Job drawing, mm, ordinate dimensions from the low corner. One solid piece. Coordinates: 2 decimals unless noted, no trailing zeros. Order: outer loops, then holes, each group sorted by start corner. A loop starts at its lowest first (then second) coordinate and runs counter-clockwise, first axis right, second up. Notation, with made-up numbers: M -16.5,18 L 33.5,18 A20 ccw 33.5,49 Z; hole C 58,-9.75 d7. An arc over 180 degrees is marked long. Write item = value, one per line.
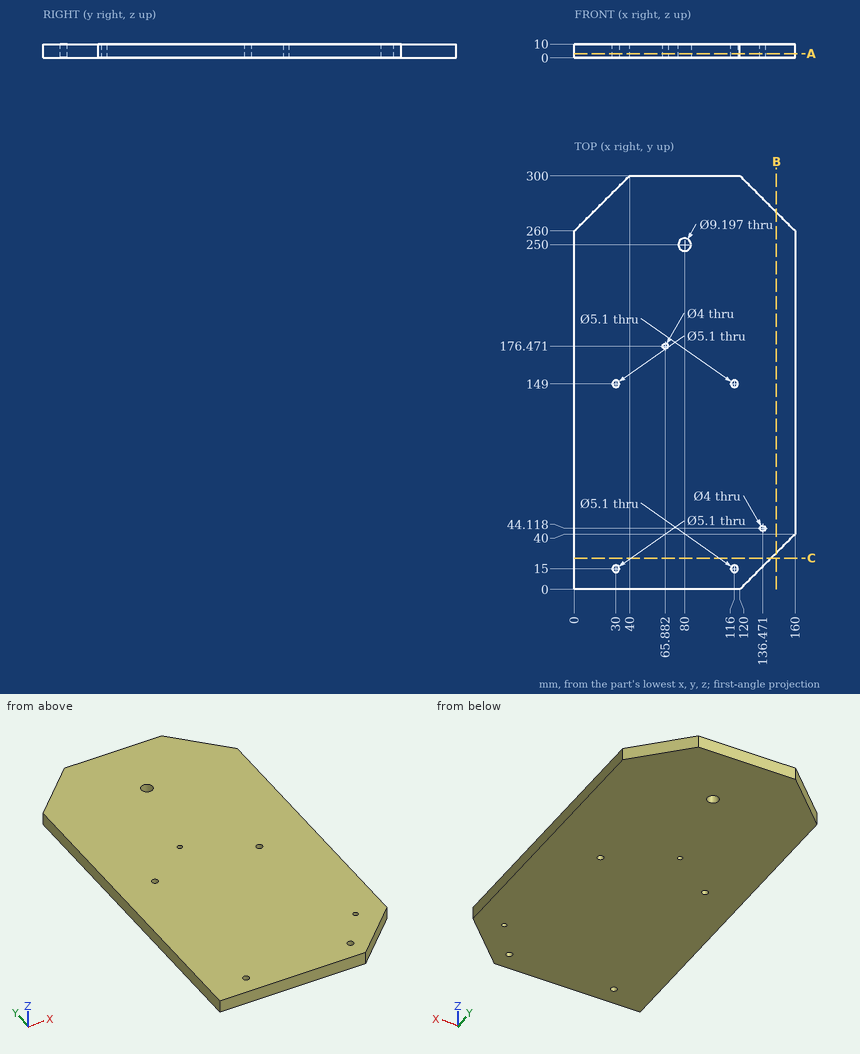
(1) Slice it at B-B, the plane x = 146.5. Write the cut outline in (y, z), then the cut area to 3 significant figures.
Evaluation:
outline = M 26.5,0 L 273.5,0 L 273.5,10 L 26.5,10 Z
area = 2,470 mm²
(2) Slice it at A-A, the plane z = 3. Write the cut outline in (x, y).
Evaluation:
outline = M 0,0 L 120,0 L 160,40 L 160,260 L 120,300 L 40,300 L 0,260 Z; hole C 30,15 d5.1; hole C 30,149 d5.1; hole C 65.88,176.47 d4; hole C 80,250 d9.2; hole C 116,15 d5.1; hole C 116,149 d5.1; hole C 136.47,44.12 d4
(3) Slice it at C-C, the plane y = 22.5. Write the cut outline in (x, z), then the cut area to 4 significant figures.
Evaluation:
outline = M 0,0 L 142.5,0 L 142.5,10 L 0,10 Z
area = 1,425 mm²
(4) Wall check: line 1 (Y direction, x = 116, z = 6.25); line 2 (Y direction, x = 29.5, z = 5.5); line 3 (X direction, y = 44.5, z = 3.5). Give the ranges that are in metal, low to high. Write a range as from..to.
Evaluation:
line_1 = 0..12.45, 17.55..146.45, 151.55..300
line_2 = 0..12.5, 17.5..146.5, 151.5..289.5
line_3 = 0..134.51, 138.43..160
(5) Pin check, flat tip, straight feed: pin 1 Ø3 at (x, z) = (21, 1) entering from +Y. Stop position of the tip, or through.
Evaluation:
pin_1 = 282.5
